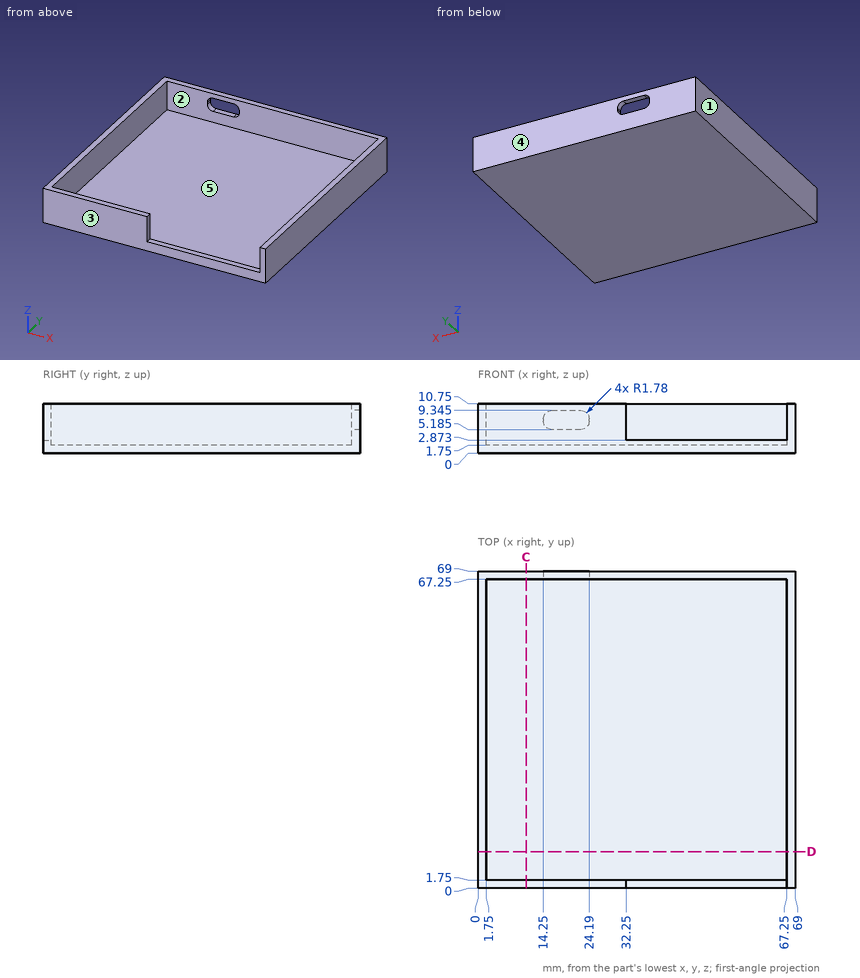
Job drawing, mm, ordinate dimensions from the low corner. One solid piece. A direction names the side the tool comes from. Give positions to 0.01 mm unless a question says otherwise; leave off trailing zeros. Loops run counter-clockwise (first coordinate to the right, second up) from the corner with the lowest first, then second, coordinate; pieces in that order, holes last. Notation, with made-up numbers: M 64,-36 L 114,-36 A19 cw 114,-20 Z; hole C 53.25,24.5 d5. An arc over 180 degrees is marked long. Use one line per item in the form item = value.
Item 1: Flat gauge pins, fed straight in: pin 1 Ø19.5 at (x, y) = (22.5, 31.5) entering from +Z; pin 2 Ø0.9 at (x, y) = (41.5, 1) entering from +Z. Where does each tip first touch, or does it go through?
Filled in:
pin_1 = 1.75
pin_2 = 2.87
Item 2: Two-plate mould, pull along Y, no slides. Class the marked faces 1, 2 and 3: released by +Y, released by -Y, zero draft, split by the parting line, or undercut.
Filled in:
face_1 = zero draft
face_2 = undercut
face_3 = released by -Y
Item 3: Drill centre lines: L1, parallel to X at y = 19, z = 4.5; L2, parallel to Y at x = 37.5, z = 8.75. Where is each one in solid material? Low to high.
Filled in:
L1 = 0 to 1.75, 67.25 to 69
L2 = 67.25 to 69
Item 4: Slice it at C-C on x = 10.5. List the corners of the cut face in (y, z).
Filled in:
outline = M 0,0 L 69,0 L 69,10.75 L 67.25,10.75 L 67.25,1.75 L 1.75,1.75 L 1.75,10.75 L 0,10.75 Z
Item 5: Which spindle directions (+Z, -Z, +X, -X, +Y, -Y) get a long thin tool onto all of the face, cutting with end or side? Do the marked faces 4 and 5. Say none if no direction does.
Filled in:
face_4 = +Z, -Z, +X, -X, +Y
face_5 = +Z
